Here's how the part is built. I have some questions about the finished solid (model axes, mm). Give positions to 0.01 mm unless a question says otherwise; leave off trailing zeros. Loops run counter-clockwise (first coordinate to the right, second up) from the corner with the lowest first, then second, coordinate; pieces in that order, holes last. Notation, with made-up numbers: (83.25, 12) - (93.25, 12) arc R24 ccw to (93.25, 43) - close; hole circle Ø1 at (65.25, 63.5). An arc over 180 degrees is marked (long way). Return JSON: item names as keys, results as strings. Group by question number.
(1) If we section it at A-A (z = 0): Please give me the cut outline in (x, y), then the cut area to 3 significant figures.
(2) For P1, Ø3.5, axis at y = 9.5, z = 3.33, coming from the -X side, with a flat end and sliding along its axis, tell me the tip position at first contact or that it passes through.
(3) If we section it at C-C (x = 3.3): State how many separate pieces and enclosed holes the cut face has, then the cut area to 3 significant figures.
(4) If we section it at D-D (y = 25): Please give me the cut outline in (x, z).
(5) If we section it at B-B (y = 8.5): Please give me the cut outline in (x, z).
(6) I need wall thicknesses on probe 1 along Y at (x, z) = (4, -9); probe 2 along Y at (x, z) = (2.4, 0); probe 3 along Y at (x, z) = (0.55, 18). Which ranges of each line are inside material? Lowest first, please. Write a range as [from, to].
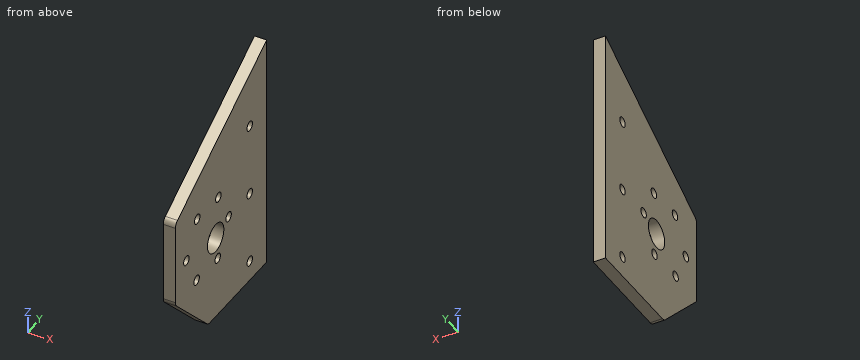
```python
from build123d import *

# Parameters (mm, degrees)
SKETCH1_R           = 6
SKETCH1_R_2         = 2
BOSS_EXTRUDE1_DEPTH = 5


with BuildPart() as part:
    # Sketch1 → Boss-Extrude1 (new body)
    with BuildSketch(Plane(origin=(0, 0, 0), x_dir=(0, 0, -1), z_dir=(1, 0, 0))):
        with BuildLine():
            Line((34.894448725, 36.555579518), (34.894448725, -4.257359313))
            ThreePointArc((34.894448725, -4.257359313), (34.666087322, -5.40540961), (34.015769068, -6.378679656))
            Line((34.015769068, -6.378679656), (11.773128381, -28.621320344))
            ThreePointArc((11.773128381, -28.621320344), (10.799858335, -29.271638598), (9.651808037, -29.5))
            Line((9.651808037, -29.5), (-23.373500468, -29.5))
            ThreePointArc((-23.373500468, -29.5), (-24.873500468, -29.098076211), (-25.971576679, -28))
            Line((-25.971576679, -28), (-63.788019311, 37.5))
            Line((-63.788019311, 37.5), (34.894448725, 37.5))
            Line((34.894448725, 37.5), (34.894448725, 36.555579518))
        make_face()
        Circle(SKETCH1_R, mode=Mode.SUBTRACT)
        with Locations((9.68016301, -13.983720681)):
            Circle(SKETCH1_R_2, mode=Mode.SUBTRACT)
        with Locations((-3.876799059, -21.49762642)):
            Circle(SKETCH1_R_2, mode=Mode.SUBTRACT)
        with Locations((-17.162513345, -13.513905738)):
            Circle(SKETCH1_R_2, mode=Mode.SUBTRACT)
        with Locations((-16.891265561, 1.983720681)):
            Circle(SKETCH1_R_2, mode=Mode.SUBTRACT)
        with Locations((-3.334303492, 9.49762642)):
            Circle(SKETCH1_R_2, mode=Mode.SUBTRACT)
        with Locations((9.951410794, 1.513905738)):
            Circle(SKETCH1_R_2, mode=Mode.SUBTRACT)
        with Locations((-3.605551275, 25)):
            Circle(SKETCH1_R_2, mode=Mode.SUBTRACT)
        with Locations((26.394448725, 25)):
            Circle(SKETCH1_R_2, mode=Mode.SUBTRACT)
        with Locations((-33.605551275, 25)):
            Circle(SKETCH1_R_2, mode=Mode.SUBTRACT)
    extrude(amount=BOSS_EXTRUDE1_DEPTH)


solid = part.part
```
Values:
{
 "1": {"outline": "(0, -29.5) - (5, -29.5) - (5, -6) - (0, -6) - close; (0, 6) - (5, 6) - (5, 37.5) - (0, 37.5) - close", "area": "275 mm2"},
 "2": {"P1": "through"},
 "3": {"separate pieces": "1", "enclosed holes": "10", "area": "4,800 mm2"},
 "4": {"outline": "(0, -34.89) - (5, -34.89) - (5, -28.39) - (0, -28.39) - close; (0, -24.39) - (5, -24.39) - (5, 1.61) - (0, 1.61) - close; (0, 5.61) - (5, 5.61) - (5, 31.61) - (0, 31.61) - close; (0, 35.61) - (5, 35.61) - (5, 56.57) - (0, 56.57) - close"},
 "5": {"outline": "(0, -34.89) - (5, -34.89) - (5, 1.6) - (0, 1.6) - close; (0, 5.07) - (5, 5.07) - (5, 47.04) - (0, 47.04) - close"},
 "6": {"probe 1": "[-29.5, -15.86], [-12.1, -0.25], [3.27, 37.5]", "probe 2": "[-29.5, -6], [6, 37.5]", "probe 3": "[-29.5, -15.33], [-11.7, 0.32], [3.65, 37.5]"}
}
